Autodesk Inventor part; units mm, degrees
ref_plane "Work Plane1" through (2.75, 0, 0) normal (0, -1, 0) x (1, 0, 0)
ref_plane "YZ Plane" through (0, 0, 0) normal (1, 0, 0) x (0, 1, 0)
ref_plane "XZ Plane" through (0, 0, 0) normal (0, 1, 0) x (-1, 0, 0)
sketch "Schizzo1" plane through (0, 0, 0) normal (0, 0, 1) x (1, 0, 0)
  line L0 (35, 4) -> (35, 0)
  line L1 (-35, 0) -> (35, 0)
  line L2 (-49, 0) -> (49, 0)
  line L3 (0, 4.8) -> (0, -0.8)
  line L4 (-35, 4) -> (-35, 0)
  line L5 (0, 4) -> (0, 0) construction
  line L6 (-49, 0) -> (49, 0)
  line L7 (-35, 4) -> (35, 4)
  dimension "d13" = 8
  dimension "d87" = 70
  dimension "d88" = 35
revolve "Corpo" add sketch "Schizzo1" angle 360 about axis through (-35, 0, 0) along (1, 0, 0)
thread "Filettatura1"
chamfer "Smusso1" distance 0.864 angle 45 1 edges at (35, -4, 0) measured on face at (11.6667, 3.987, -0.3219)
chamfer "Smusso2" distance 0.864 angle 45 1 edges at (-35, -4, 0) measured on face at (11.0907, 3.987, -0.3219)
ref_plane "Work Plane1" through (2.75, 0, 0) normal (0, -1, 0) x (1, 0, 0)
equation "\"d13\" = NND"
equation "\"d87\" = NLG"
equation "\"d88\" = 0.5 * NLG"
equation "\"d1\" = GEL"
equation "\"d9\" = -0.5 * SPD + 0.5 * NND"
equation "\"d10\" = -0.5 * SPD + 0.5 * NND"
equation "\"d11\" = -0.5 * SPD + 0.5 * NND"
equation "\"d12\" = -0.5 * SPD + 0.5 * NND"
equation "\"NLG\" = 70"
equation "\"GEL\" = NLG"
equation "\"GAL\" = 0.61345 * PTC"
equation "\"SPD\" = 6.272"
equation "\"d0\" = NND"
equation "\"GUL\" = 0.61345 * PTC"
equation "\"NND\" = 8"
equation "\"GUL1\" = GUL"
equation "\"GAL1\" = GAL"
equation "\"d80\" = -GUL - GEL"
equation "\"d86\" = -GEL + GUL1"
equation "\"PTC\" = 1.25"
equation "\"THREADDIA\" = 8"
equation "\"TOA\" = 30deg"
equation "\"GD1\" = THREADDIA - 1.2269 * PTC"
properties part number "DIN 976-1 - M8 x 70 - B" material "Acciaio, Dolce"
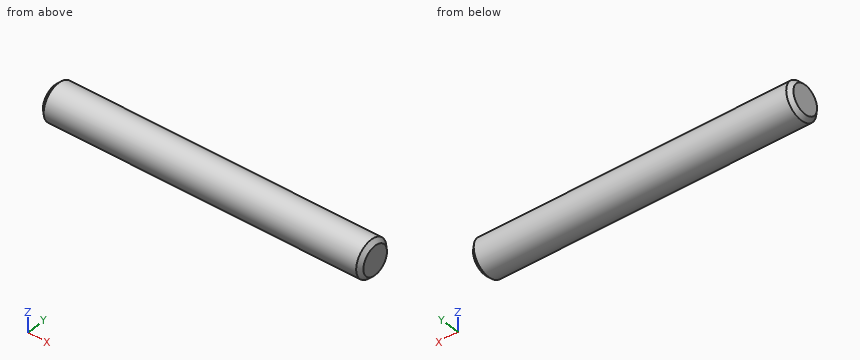
Verification items for the finished model (mm, model axes). Coordinates: 2 decimals unless noted, no trailing zeros. Write each loop counter-clockwise with the first axis right and the second up, starting at its lowest first coordinate (ties: lowest second). Pieces come first, ordered by that corner, then holes. Notation, with made-up numbers: (-13.75, 29) - (18.25, 29) arc R21 cw to (18.25, 62) - close; hole circle Ø11 at (-33, 3). An arc over 180 degrees is marked (long way). One line per question, with ' | ' between items. Start each with the question number.
1. Material ranges on line 1 along Y through (x, z) = (28, 2.5); line 2 along Z through (x, y) = (-26.5, -0.25), recorded low to high.
2. Gauge pin test, flat ends, axial feed: P1, Ø4, axis at x = 24, z = -2.5, coming from the +Y side; P2, Ø1, axis at x = -21, y = 1, coming from the -Z side. Record the tip position at first contact, or that the pin passes through.
3. Section check A-A (x = 30). Enter the section's corners in (y, z), plus the area to 3 significant figures.
Computed values:
1) line 1: -3.12 to 3.12 | line 2: -3.99 to 3.99
2) P1: y = 3.97 | P2: z = -3.97
3) outline: circle Ø8 at (0, 0) | area: 50.3 mm²
